from build123d import *

# Parameters (mm, degrees)
F0_W     = 140
F0_H     = 70
F1_DEPTH = 7
F2_W     = 8
F2_H     = 8
F3_DEPTH = 50
F5_DEPTH = 8
F6_R     = 10
F7_R     = 5
F9_R     = 2


with BuildPart() as f1:
    # F0 (on Top) → F1 (new body)
    with BuildSketch(Plane.XY):
        Rectangle(F0_W, F0_H)
    extrude(amount=F1_DEPTH)

    # F2 (on face) → F3 (join)
    with BuildSketch(Plane.XY.offset(7)):
        with Locations((26, 0)):
            Rectangle(F2_W, F2_H)
    extrude(amount=F3_DEPTH)

    # F6
    f6_edges = [f1.edges().sort_by_distance(p)[0] for p in [
        (-70, 35, 3.5),
        (-70, -35, 3.5),
        (70, 35, 3.5),
        (70, -35, 3.5),
    ]]
    fillet(f6_edges, radius=F6_R)

    # F7
    f7_edges = [f1.edges().sort_by_distance(p)[0] for p in [
        (0, -35, 7),
        (70, 0, 7),
        (0, 35, 7),
        (-70, 0, 7),
    ]]
    fillet(f7_edges, radius=F7_R)


with BuildPart() as f5:
    # F4 (on face) → F5 (new body)
    with BuildSketch(Plane.YZ.offset(30)):
        Polygon((-14.606602, 67.606602), (-4, 57), (4, 57), (14.606602, 67.606602), (10.606602, 71.606602), (0, 61), (-10.606602, 71.606602), align=None)
    extrude(amount=-F5_DEPTH)


with BuildPart() as f1_1:
    add(f1.part)

    # F8: union F5
    add(f5.part)

    # F9
    f9_edges = [f1_1.edges().sort_by_distance(p)[0] for p in [
        (30, 9.303301, 62.303301),
        (30, 4, 32),
        (30, 5.303301, 66.303301),
        (30, -5.303301, 66.303301),
        (30, -9.303301, 62.303301),
        (30, -4, 32),
        (26, 10.606602, 71.606602),
        (26, -10.606602, 71.606602),
        (26, 0, 61),
        (26, 14.606602, 67.606602),
        (30, -12.606602, 69.606602),
        (30, 12.606602, 69.606602),
        (22, 12.606602, 69.606602),
        (22, -5.303301, 66.303301),
        (26, -4, 57),
        (26, -4, 7),
        (22, -4, 32),
        (22, -9.303301, 62.303301),
        (26, -14.606602, 67.606602),
        (22, -12.606602, 69.606602),
        (22, 5.303301, 66.303301),
        (22, 9.303301, 62.303301),
        (22, 4, 32),
        (26, 4, 57),
        (26, 4, 7),
        (22, 0, 7),
        (30, 0, 7),
    ]]
    fillet(f9_edges, radius=F9_R)


solid = f1_1.part
Verification items for the finished model (mm, model axes). A direction names the side the tool comes from. Coordinates: 2 decimals unless noted, no trailing zeros. Write each loop counter-clockwise with the first axis right and the second up, starting at its lowest first coordinate (ties: lowest second). Pieces come first, ordered by that corner, then holes. Notation, with made-up numbers: M 1,59.25 L 25,59.25 A24 ccw 25,95.25 Z; hole C 30.5,86 d6. An arc over 180 degrees is marked long. Use a Markdown table: item, result.
Q1. Sectioned sample at C-C, the plane x = 14. Record the boundary of the cut face in (y, z), plus the area to 3 significant figures.
Reply:
| item | result |
|---|---|
| outline | M -35,0 L 35,0 L 35,2 A5 ccw 30,7 L -30,7 A5 ccw -35,2 Z |
| area | 479 mm² |
Q2. Set-up check for faces 4 (the face through (29.43, 8.52, 62.37)), 5 (the face through (26, -9, 62)), 6 (the face through (30, 0, 39)): record each of +Z, -Z, +X, -X, +Y, -Y from which the full face is reachable in a straight line by a thin tool's end or side.
Reply:
| item | result |
|---|---|
| face 4 | +X, +Y |
| face 5 | +X, -X, -Y |
| face 6 | +Z, +X, +Y, -Y |
Q3. Sectioned sample at A-A, the plane z = 27. Record the boundary of the cut face in (x, y).
Reply:
| item | result |
|---|---|
| outline | M 22,-2 A2 ccw 24,-4 L 28,-4 A2 ccw 30,-2 L 30,2 A2 ccw 28,4 L 24,4 A2 ccw 22,2 Z |
Q4. Go/stop test with flat-tipped pins: P1, Ø8, axis at x = -23, y = -12.5, coming from the +Z side; P2, Ø19, axis at y = -6, z = 37, coming from the -X side; P3, Ø3, axis at x = 26.5, z = 41, coming from the +Y side. Record where each tip stops, or that it passes through.
Reply:
| item | result |
|---|---|
| P1 | stops at z = 7 |
| P2 | stops at x = 22 |
| P3 | stops at y = 4 |
Q5. Sectioned sample at B-B, the plane y = -19. Record the boundary of the cut face in (x, z), plus the area to 3 significant figures.
Reply:
| item | result |
|---|---|
| outline | M -70,0 L 70,0 L 70,2 A5 ccw 65,7 L -65,7 A5 ccw -70,2 Z |
| area | 969 mm² |
Q6. Draft check along Z on faces 1 (the face through (1, -33, 6)), 2 (the face through (29.399, -8.426, 62.232)), 3 (the face through (22, 0, 39)). Enter one of: +Z half, -Z half, draft (parallel to the pull), parting line (faces both ways), or undercut.
Reply:
| item | result |
|---|---|
| face 1 | +Z half |
| face 2 | undercut |
| face 3 | draft |
Q7. Thickness scan on line 1 (Z direction, x = 36.5, y = 0.5). Record the ranges inside material, lowest first.
Reply:
| item | result |
|---|---|
| line 1 | z = 0 to 7 |
